```python
from build123d import *

# Parameters (mm, degrees)
FILETE1_R = 1


with BuildPart() as part:
    # Esboço1 → Revolução1 (revolve)
    with BuildSketch(Plane.XY):
        Polygon((0, 0), (0, 4.3), (5, 4.3), (5, 4.7), (7, 4.7), (13, 3), (13, 0), align=None)
    revolve(axis=Axis((13, 0, 0), (-1, 0, 0)))

    # Filete1
    filete1_edges = [part.edges().sort_by_distance(p)[0] for p in [
        (0, -4.3, 0),
    ]]
    fillet(filete1_edges, radius=FILETE1_R)


solid = part.part
```
For this review, take the finished solid that the model builds, in its own axes (mm). A direction names the side the tool comes from. Round coordinates to 2 decimals unless told otherwise and drop trailing zeros. Write each loop counter-clockwise with the first axis right and the second up, starting at its lowest first coordinate (ties: lowest second). Pieces come first, ordered by that corner, then holes. Notation, with made-up numbers: (5.5, 53) -> (37.5, 53) arc R11 cw to (37.5, 65) -> close; hole circle Ø1 at (56, 53). An arc over 180 degrees is marked (long way). One line per question, with ' | ' between items. Start each with the question number.
(1) Tool access review of faces 1 (the face through (5, -2, 4)), 2 (the face through (13, 0, 0)): name each direction out of +Z, -Z, +X, -X, +Y, -Y from which nothing blocks a thin tool from reaching the whole face with its end or side.
(2) Add section C-C, the plane x = 3. Write out the cut boundary in (y, z), plus the area to 3 significant figures.
(3) For line 1 along Y through (x, z) = (1, 0); line 2 along Y through (x, z) = (10.5, 3); line 3 along Z through (x, y) = (7, -3.25), list the stretches that pass through material, from the lowest coordinate up. Write a range as from..to.
(4) Add section A-A, the plane y = 0. Write out the cut boundary in (x, z).
(5) Add section B-B, the plane x = 6. Write out the cut boundary in (y, z).
(6) Insertion check: P1, Ø1.5, axis at x = 1.5, z = 3, coming from the -Y side; P2, Ø1, axis at x = 4, z = 2, coming from the +Y side; P3, Ø5, axis at x = 10, y = -0.5, coming from the +Z side. Each pin has a flat end and moves straight along its axis. Give the tip position at first contact, or say it passes through.
Answer list:
1) face 1: -X | face 2: +Z, -Z, +X, +Y, -Y
2) outline: circle Ø8.6 at (0, 0) | area: 58.1 mm²
3) line 1: -4.3..4.3 | line 2: -2.18..2.18 | line 3: -3.4..3.4
4) outline: (0, -3.3) arc R1 ccw to (1, -4.3) -> (5, -4.3) -> (5, -4.7) -> (7, -4.7) -> (13, -3) -> (13, 3) -> (7, 4.7) -> (5, 4.7) -> (5, 4.3) -> (1, 4.3) arc R1 ccw to (0, 3.3) -> close
5) outline: circle Ø9.4 at (0, 0)
6) P1: y = -3.66 | P2: y = 4.03 | P3: z = 4.55
